Study the drawing (mm; zero at the part's minimum x, y, z) and answer. A direction names the side the tool comes from. Round coordinates to 2 decimals unless told otherwise and drop trailing zeros. Loops run counter-clockwise (first coordinate to the right, second up) from the corner with the lowest first, then second, coordinate; pieces in that order, holes last. Notation, with made-up numbers: M 68,40.5 L 127,40.5 A13 cw 127,62.5 Z; hole C 89,67 d4. An arc over 180 degrees is marked long. Write each question's results on one line, items separated by ' | '.
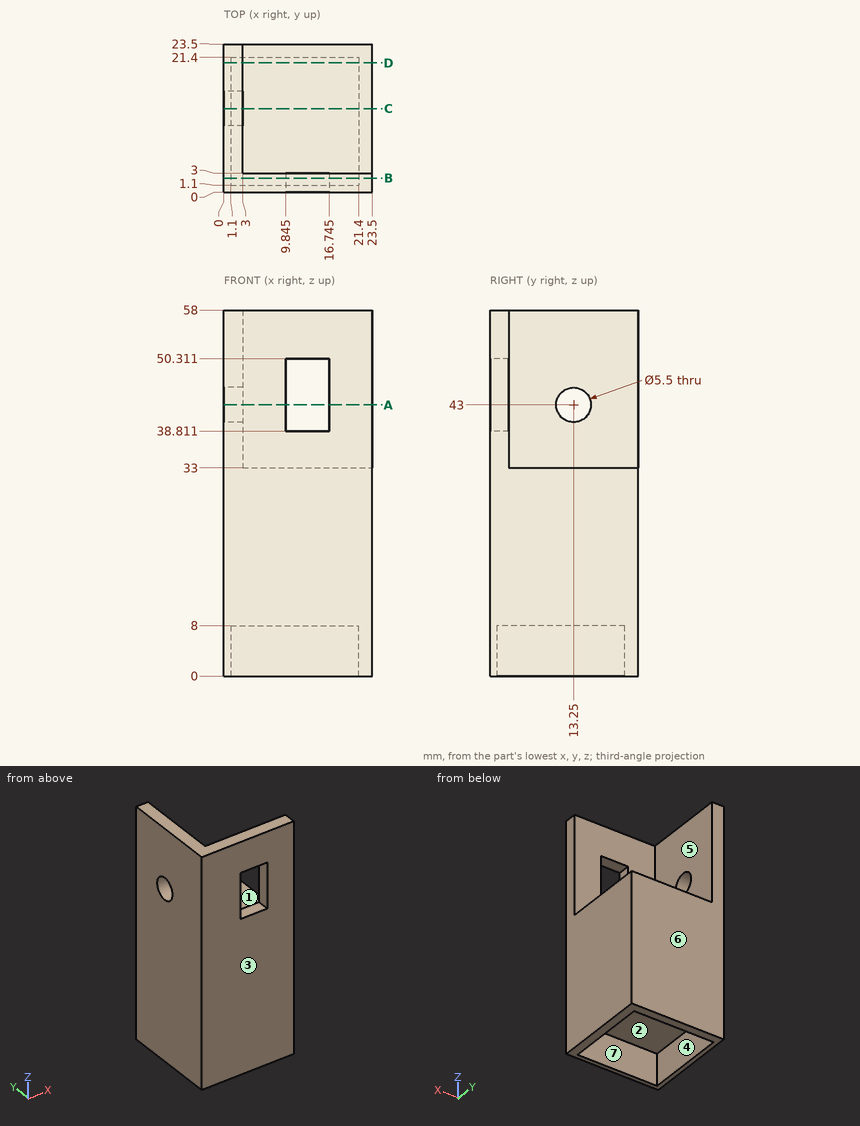
Item 1: The part is cut by section C-C (y = 13.25). Determine the outline of the cut face in (x, z), plus the area to 3 significant figures.
Outcome:
outline: M 0,0 L 1.1,0 L 1.1,8 L 21.4,8 L 21.4,0 L 23.5,0 L 23.5,33 L 3,33 L 3,40.25 L 0,40.25 Z; M 0,45.75 L 3,45.75 L 3,58 L 0,58 Z | area: 672 mm2
Item 2: The mould has two halves that part along Y. Classify the marked faces 4, 5, 6 and 7: pulls with the +Y half, pulls with the -Y half, needs draft (parallel to the pull), parting line crosses it, or undercut.
Outcome:
face 4: undercut | face 5: needs draft | face 6: pulls with the +Y half | face 7: undercut
Item 3: Straight lines are drawn through the part: line 1 (X direction, y = 14, z = 4.5); line 2 (Z direction, x = 1.65, y = 13.25); line 3 (Z direction, x = 7.75, y = 18.5). For each, find the intervals that lie inside material, in ascending order.
Outcome:
line 1: x = 0 to 1.1, 21.4 to 23.5 | line 2: z = 8 to 40.25, 45.75 to 58 | line 3: z = 8 to 33
Item 4: The part is cut by section A-A (z = 43). Determine the outline of the cut face in (x, y) (1 decimal), plus the area to 3 significant figures.
Outcome:
outline: M 0,0 L 9.8,0 L 9.8,3 L 3,3 L 3,10.5 L 0,10.5 Z; M 0,16 L 3,16 L 3,23.5 L 0,23.5 Z; M 16.7,0 L 23.5,0 L 23.5,3 L 16.7,3 Z | area: 94.8 mm2
Item 5: For the marked faces 1, 2 and 3, determine the directions among +Z, -Z, +X, -X, +Y, -Y from which every point of the face is accessible in a straight line to the end or side of a thin tool.
Outcome:
face 1: +Z, +X, +Y | face 2: -Z | face 3: +Z, -Z, +X, -X, -Y
Item 6: The part is cut by section B-B (y = 2.25). Determine the outline of the cut face in (x, z) (1 decimal).
Outcome:
outline: M 0,0 L 1.1,0 L 1.1,8 L 21.4,8 L 21.4,0 L 23.5,0 L 23.5,58 L 0,58 Z; hole M 9.8,38.8 L 16.7,38.8 L 16.7,50.3 L 9.8,50.3 Z
Item 7: The part is cut by section D-D (y = 20.5). Determine the outline of the cut face in (x, z), plus the area to 3 significant figures.
Outcome:
outline: M 0,0 L 1.1,0 L 1.1,8 L 21.4,8 L 21.4,0 L 23.5,0 L 23.5,33 L 3,33 L 3,58 L 0,58 Z | area: 688 mm2
Item 8: Flat-ended cylindrical pins translate along their axes: pin 1 (1 mm diameter, centred on x = 9.5, z = 45.5, fed in from +Y); pin 2 (4.5 mm diameter, centred on y = 13.25, z = 43, fed in from -X); pin 3 (6 mm diameter, centred on x = 10.5, y = 8.5, fed in from -Z); pin 4 (8 mm diameter, centred on x = 9, y = 14.5, fed in from +Z). Find the tip coordinate at first contact, or state that the pin passes through.
Outcome:
pin 1: stops at y = 3 | pin 2: passes through | pin 3: stops at z = 8 | pin 4: stops at z = 33
